Here's how the part is built. I have some questions about the finished solid (model axes, mm). Face numbers are marked on the shaded views. A direction names the side the tool comes from. Coordinates: 2 decimals unless noted, no trailing zeros. Loops run counter-clockwise (first coordinate to the right, second up) from the corner with the lowest first, then second, coordinate; pieces in that order, holes last. Notation, with made-up numbers: (14, 12.25) - (49, 12.25) arc R10 ccw to (49, 18.25) - close; hole circle Ø9 at (-27, 89.25). An arc over 180 degrees is marked (long way). Use a Markdown table: item, result.
```python
from build123d import *

# Parameters (mm, degrees)
SKETCH1_W           = 31.75
SKETCH1_H           = 57.15
BOSS_EXTRUDE1_DEPTH = 2.286
SKETCH2_W           = 31.75
SKETCH2_H           = 57.15
SKETCH2_W_2         = 27.686
SKETCH2_H_2         = 53.086
BOSS_EXTRUDE2_DEPTH = 12.7
SKETCH3_R           = 1.27
CUT_EXTRUDE1_DEPTH  = 36.06902123
SKETCH4_W           = 16.51
SKETCH4_H           = 7.874
CUT_EXTRUDE2_DEPTH  = 46.267795628


with BuildPart() as part:
    # Sketch1 → Boss-Extrude1 (new body)
    with BuildSketch(Plane(origin=(0, 0, 0), x_dir=(1, 0, 0), z_dir=(0, 1, 0))):
        Rectangle(SKETCH1_W, SKETCH1_H)
    extrude(amount=BOSS_EXTRUDE1_DEPTH)

    # Sketch2 → Boss-Extrude2 (add)
    with BuildSketch(Plane(origin=(0, 2.286, 0), x_dir=(1, 0, 0), z_dir=(0, 1, 0))):
        Rectangle(SKETCH2_W, SKETCH2_H)
        Rectangle(SKETCH2_W_2, SKETCH2_H_2, mode=Mode.SUBTRACT)
    extrude(amount=BOSS_EXTRUDE2_DEPTH)

    # Sketch3 → Cut-Extrude1 (cut, through all)
    with BuildSketch(Plane(origin=(0, 2.286, 0), x_dir=(1, 0, 0), z_dir=(0, 1, 0))):
        with Locations(Location((-0.127, 16.383, 0), (0, 0, 270))):
            Circle(SKETCH3_R)
        with Locations(Location((-0.127, 10.795, 0), (0, 0, 270))):
            Circle(SKETCH3_R)
        with Locations(Location((-0.127, 5.207, 0), (0, 0, 270))):
            Circle(SKETCH3_R)
        with Locations(Location((0, -0.381, 0), (0, 0, 270))):
            Circle(SKETCH3_R)
        with Locations(Location((0, -9.176980695, 0), (0, 0, 270))):
            Circle(SKETCH3_R)
    extrude(amount=-CUT_EXTRUDE1_DEPTH, mode=Mode.SUBTRACT)

    # Sketch4 → Cut-Extrude2 (cut, through all)
    with BuildSketch(Plane.ZY.offset(15.875)):
        with Locations((0, 11.049)):
            Rectangle(SKETCH4_W, SKETCH4_H)
    extrude(amount=-CUT_EXTRUDE2_DEPTH, mode=Mode.SUBTRACT)


solid = part.part
```
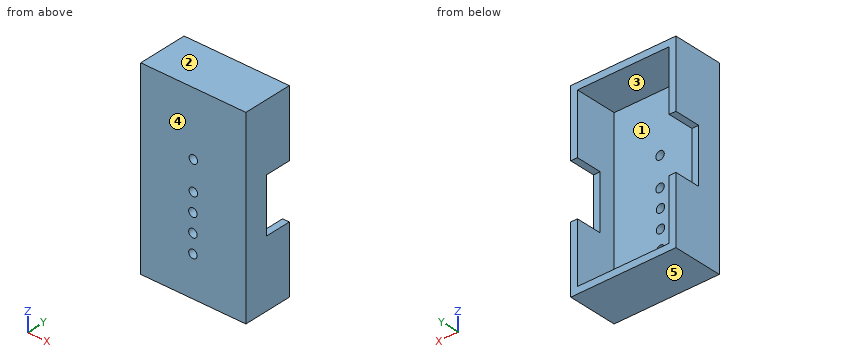
Q1. I want a section at B-B, the plane y = 3.5. Write out the boundary of the cut face in (x, z) (3 decimals).
Check values:
| item | result |
|---|---|
| outline | (-15.875, -28.575) - (15.875, -28.575) - (15.875, 28.575) - (-15.875, 28.575) - close; hole (-13.843, -26.543) - (13.843, -26.543) - (13.843, 26.543) - (-13.843, 26.543) - close |
Q2. Please list where these lines run through material, in increasing order: L1, parallel to Z at x = -12.5, y = 9.25 (3 decimals); L2, parallel to X at y = 6, z = -13.5 (3 decimals); L3, parallel to Y at x = -11.5, z = -3. Write a range as from..to.
Check values:
| item | result |
|---|---|
| L1 | -28.575..-26.543, 26.543..28.575 |
| L2 | -15.875..-13.843, 13.843..15.875 |
| L3 | 0..2.29 |
Q3. Which directions (+Z, -Z, +X, -X, +Y, -Y) give clear straight access to the entire face, cutting with the end or side of a thin tool? Please do the marked faces 1 and 2.
Check values:
| item | result |
|---|---|
| face 1 | +Y |
| face 2 | +Z, +X, -X, +Y, -Y |
Q4. I want a section at C-C, the plane z = 1. Write out the boundary of the cut face in (x, y) (3 decimals), then the cut area to 3 significant figures.
Check values:
| item | result |
|---|---|
| outline | (-15.875, 0) - (-1.109, 0) - (-1.109, 2.286) - (-13.843, 2.286) - (-13.843, 7.112) - (-15.875, 7.112) - close; (1.109, 0) - (15.875, 0) - (15.875, 7.112) - (13.843, 7.112) - (13.843, 2.286) - (1.109, 2.286) - close |
| area | 87.1 mm^2 |
Q5. If we mould it in two halves opening along Z, with no side actions, what happens to the marked faces 3, 4 and 5? For each: pulls with the +Z half, pulls with the -Z half, needs draft (parallel to the pull), parting line crosses it, or undercut.
Check values:
| item | result |
|---|---|
| face 3 | undercut |
| face 4 | needs draft |
| face 5 | pulls with the -Z half |
Q6. I want a section at A-A, the plane y = 10.75. Write out the boundary of the cut face in (x, z) (3 decimals), then the cut area to 3 significant figures.
Check values:
| item | result |
|---|---|
| outline | (-15.875, -28.575) - (15.875, -28.575) - (15.875, -8.255) - (13.843, -8.255) - (13.843, -26.543) - (-13.843, -26.543) - (-13.843, -8.255) - (-15.875, -8.255) - close; (-15.875, 8.255) - (-13.843, 8.255) - (-13.843, 26.543) - (13.843, 26.543) - (13.843, 8.255) - (15.875, 8.255) - (15.875, 28.575) - (-15.875, 28.575) - close |
| area | 278 mm^2 |
Q7. Will these pins go through, and if not, where does the flat tip stop? P1, Ø2, axis at x = -0.5, z = 3.5, coming from the +Y side; P2, Ø1.6, axis at x = 15, z = -0.5, coming from the +Y side; P3, Ø1.5, axis at x = -0.127, z = -16.383, coming from the -Y side.
Check values:
| item | result |
|---|---|
| P1 | y = 2.29 |
| P2 | y = 7.11 |
| P3 | through |
Q8. I want a section at D-D, the plane x = 4.5. Write out the boundary of the cut face in (y, z) (3 decimals).
Check values:
| item | result |
|---|---|
| outline | (0, -28.575) - (14.986, -28.575) - (14.986, -26.543) - (2.286, -26.543) - (2.286, 26.543) - (14.986, 26.543) - (14.986, 28.575) - (0, 28.575) - close |
